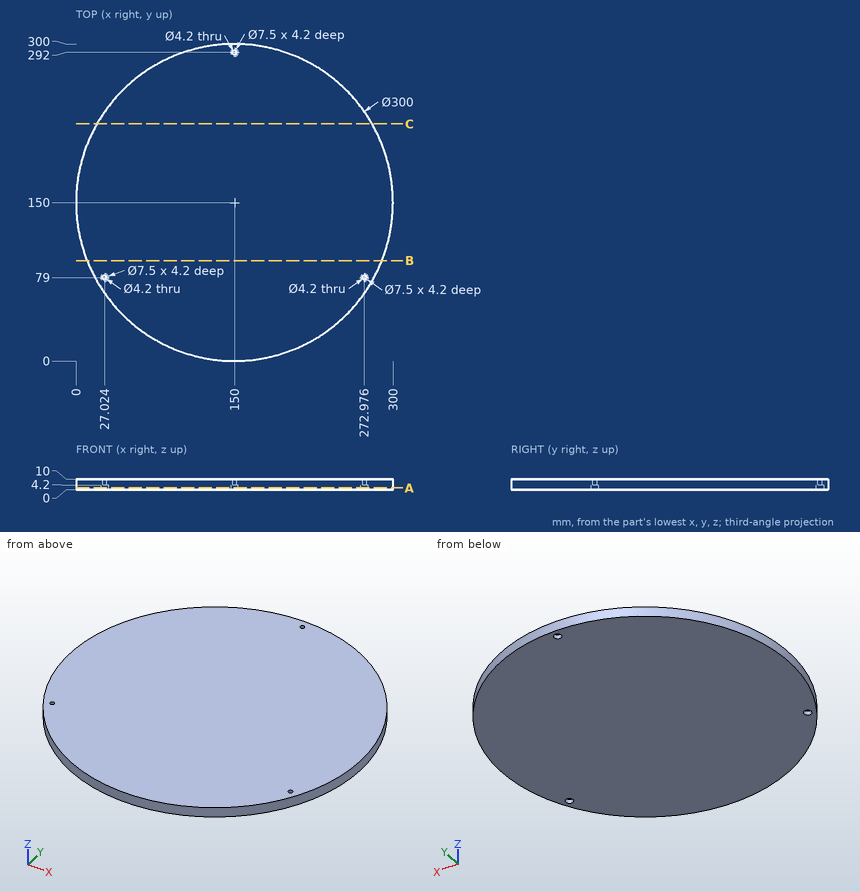
Input: dimensioned drawing with shaded views. Units: mm. Origin: part minimum x, y, z. Coordinates: 2 decimals unless noted, no trailing zeros. Loops run counter-clockwise (first coordinate to the right, second up) from the corner with the lowest first, then second, coordinate; pieces in that order, holes last.
Q1. Contact query for flat-ended pins moving along their axis: pin 1 (4 mm diameter, centred on y = 132, z = 2.5, fed in from -X); pin 2 (4 mm diameter, centred on x = 273.5, y = 80, fed in from -Z); pin 3 (1 mm diameter, centred on x = 238, z = 8.5, fed in from +Y) (1 decimal). Output: stop coordinate, or through.
Results are:
pin 1: stops at x = 0.86
pin 2: stops at z = 4.2
pin 3: stops at y = 271.8
Q2. Section B-B, the plane y = 95. Return the cut outline in (x, z), and give its area (3 significant figures).
Results are:
outline: (10.45, 0) - (289.55, 0) - (289.55, 10) - (10.45, 10) - close
area: 2,790 mm2
Q3. Section A-A, the plane z = 1.5. Give the number of separate pieces and of enclosed holes in the cut face, and give its area (3 significant figures).
Results are:
separate pieces: 1
enclosed holes: 3
area: 70,600 mm2
Q4. Line query: line 1 along Y through (x, z) = (150, 1.15); line 2 along X through (y, z) = (79, 1.5) (1 decimal); line 3 along X through (y, z) = (79, 5.65) (1 decimal). Output: solid intervals per line, ascending.
Results are:
line 1: y = 0 to 288.25, 295.75 to 300
line 2: x = 17.9 to 23.3, 30.8 to 269.2, 276.7 to 282.1
line 3: x = 17.9 to 24.9, 29.1 to 270.9, 275.1 to 282.1
Q5. Section C-C, the plane y = 224.5. Return the cut outline in (x, z), and give its area (3 significant figures).
Results are:
outline: (19.81, 0) - (280.19, 0) - (280.19, 10) - (19.81, 10) - close
area: 2,600 mm2
